Verification items for this drawing (mm, ordinates from the low corner). A direction names the side the tool comes from. Give positions to 0.01 mm unless a question says otherwise; leave off trailing zeros. Loops run counter-clockwise (first coordinate to the right, second up) from the corner with the lowest first, then second, coordinate; pieces in that order, holes last. Notation, with made-up numbers: (-39.5, 13.5) -> (12.5, 13.5) arc R17 ccw to (12.5, 24.5) -> close; hole circle Ø11 at (17, 79). An arc over 180 degrees is marked (long way). Answer as a JSON object with one key per item and string values.
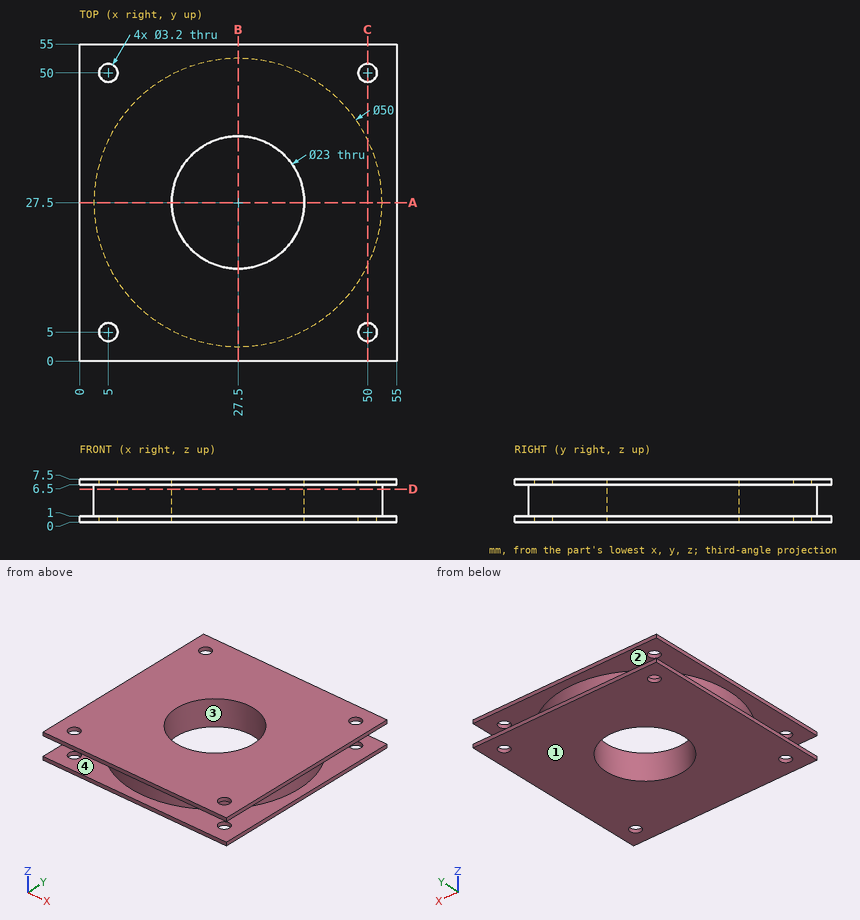
1) Depth check by flat-ended pin: P1, Ø3, axis at x = 5, y = 50, coming from the -Z side. Enter the tip coordinate at first touch or a pass-through.
Geometry check:
{"P1": "passes through"}
2) Draft check along Y on the marked faces 3 and 4. Enter one of: pulls with the +Y half, pulls with the -Y half, needs draft (parallel to the pull), parting line crosses it, or undercut.
Geometry check:
{"face 3": "undercut", "face 4": "needs draft"}
3) Section check C-C on x = 50. Record the cut outline in (y, z).
Geometry check:
{"outline": "(0, 0) -> (3.4, 0) -> (3.4, 1) -> (0, 1) -> close; (0, 6.5) -> (3.4, 6.5) -> (3.4, 7.5) -> (0, 7.5) -> close; (6.6, 0) -> (48.4, 0) -> (48.4, 1) -> (38.4, 1) -> (38.4, 6.5) -> (48.4, 6.5) -> (48.4, 7.5) -> (6.6, 7.5) -> (6.6, 6.5) -> (16.6, 6.5) -> (16.6, 1) -> (6.6, 1) -> close; (51.6, 0) -> (55, 0) -> (55, 1) -> (51.6, 1) -> close; (51.6, 6.5) -> (55, 6.5) -> (55, 7.5) -> (51.6, 7.5) -> close"}
4) Material ranges on line 1 along X through (y, z) = (50, 7.3); line 2 along Z through (x, y) = (3, 51.5), recorded low to high. Write a range as from..to.
Geometry check:
{"line 1": "x = 0..3.4, 6.6..48.4, 51.6..55", "line 2": "z = 0..1, 6.5..7.5"}
5) Tool access check on the marked faces 1 and 2. Record the directions out of +Z, -Z, +X, -X, +Y, -Y that give a thin tool (end or side, any length) a straight path to the whole face; none if there is none.
Geometry check:
{"face 1": "-Z, +X, -X, +Y, -Y", "face 2": "none"}
6) Section check A-A on y = 27.5. Record the cut outline in (x, z), plus the area to 4 significant figures.
Geometry check:
{"outline": "(0, 0) -> (16, 0) -> (16, 7.5) -> (0, 7.5) -> (0, 6.5) -> (2.5, 6.5) -> (2.5, 1) -> (0, 1) -> close; (39, 0) -> (55, 0) -> (55, 1) -> (52.5, 1) -> (52.5, 6.5) -> (55, 6.5) -> (55, 7.5) -> (39, 7.5) -> close", "area": "212.5 mm2"}
7) Section check D-D on z = 5.75. Record the cut outline in (x, y), plus the area to 3 significant figures.
Geometry check:
{"outline": "circle Ø50 at (27.5, 27.5); hole circle Ø23 at (27.5, 27.5)", "area": "1,550 mm2"}
